```python
from build123d import *

# Parameters (mm, degrees)
F0_W     = 50.8
F0_H     = 19.05
F1_DEPTH = 1111.25
F2_W     = 122.435573
F2_H     = 50.8
F2_W_2   = 93.867282
F2_W_3   = 343.160421
F2_W_4   = 175.76392
F2_W_5   = 161.28926
F3_DEPTH = 25.4
F4_R     = 4.7625
F5_DEPTH = 25.4


with BuildPart() as f1:
    # F0 (on Top) → F1 (new body)
    with BuildSketch(Plane.XY):
        Rectangle(F0_W, F0_H)
    extrude(amount=F1_DEPTH)

    # F2 (on Front) → F3 (cut)
    with BuildSketch(Plane.XZ):
        with Locations((22.446524, 25.4)):
            Rectangle(F2_W, F2_H)
        with Locations((2.720783, 755.65)):
            Rectangle(F2_W_2, F2_H)
        with Locations((-38.781822, 1085.85)):
            Rectangle(F2_W_3, F2_H)
        with Locations((-28.949343, 254)):
            Rectangle(F2_W_4, F2_H)
        with Locations((-29.98326, 482.6)):
            Rectangle(F2_W_5, F2_H)
    extrude(amount=F3_DEPTH, mode=Mode.SUBTRACT)

    # F4 (on Front) → F5 (cut)
    with BuildSketch(Plane.XZ):
        with Locations((15.875, 254)):
            Circle(F4_R)
        with Locations((15.875, 482.6)):
            Circle(F4_R)
    extrude(amount=F5_DEPTH, mode=Mode.SUBTRACT)


solid = f1.part
```
Geometry: final body of the model. Coordinates: model frame, mm. A direction names the side the tool comes from. Coordinates: 2 decimals unless noted, no trailing zeros. Order: outer loops, then holes, each group sorted by start corner. A loop starts at its lowest first (then second) coordinate and runs counter-clockwise, first axis right, second up. Notation, with made-up numbers: M 33,47 L 44,47 A19 cw 44,59 Z; hole C 41,40.5 d8. An arc over 180 degrees is marked long. Answer as CSV lines item,"result".
Q1. First-contact query: P1, Ø5, axis at x = -6, y = -3.5, coming from the +Z side; P2, Ø3, axis at x = -4.5, y = -6, coming from the -Z side; P3, Ø15, axis at x = 9, z = 482, coming from the -Y side. Flat tips, straight axial feed; report the tip coordinate or a pass-through.
Answers:
P1,"stops at z = 1060.45"
P2,"stops at z = 50.8"
P3,"stops at y = 0"
Q2. Section B-B on x = 5.5. Return the cut outline in (y, z) (3 decimals).
Answers:
outline,"M -9.525,50.8 L 0,50.8 L 0,0 L 9.525,0 L 9.525,1111.25 L 0,1111.25 L 0,1060.45 L -9.525,1060.45 L -9.525,781.05 L 0,781.05 L 0,730.25 L -9.525,730.25 L -9.525,508 L 0,508 L 0,457.2 L -9.525,457.2 L -9.525,279.4 L 0,279.4 L 0,228.6 L -9.525,228.6 Z"
Q3. Section A-A on y = -3. Return the cut outline in (x, z), and give its area (3 significant figures).
Answers:
outline,"M -25.4,50.8 L 25.4,50.8 L 25.4,228.6 L -25.4,228.6 Z; M -25.4,279.4 L 25.4,279.4 L 25.4,457.2 L -25.4,457.2 Z; M -25.4,508 L 25.4,508 L 25.4,730.25 L -25.4,730.25 Z; M -25.4,781.05 L 25.4,781.05 L 25.4,1060.45 L -25.4,1060.45 Z"
area,"43,500 mm^2"
Q4. Draft query along Z for faces 1 (the flat face through (0, -9.525, 138)), 2 (the flat face through (0, 0, 756)). Return one class per face: pulls with the +Z half, pulls with the -Z half, needs draft (parallel to the pull), parting line crosses it, or undercut.
Answers:
face 1,"needs draft"
face 2,"undercut"
Q5. Set-up query: faces 3 (the flat face through (0, 0, 483)), 4 (the flat face through (0, 0, 26)), 5 (the flat face through (0, 0, 1086)), 6 (the flat face through (-25.4, 0, 548)), 7 (the flat face through (0, -9.525, 367)). Return all of +Z, -Z, +X, -X, +Y, -Y with unobstructed straight access to the full face (end or side cutting, diameter ignored); none if empty.
Answers:
face 3,"+X, -X, -Y"
face 4,"-Z, +X, -X, -Y"
face 5,"+Z, +X, -X, -Y"
face 6,"+Z, -Z, -X, +Y, -Y"
face 7,"+Z, -Z, +X, -X, -Y"
Q6. Section C-C on z = 262. Return the cut outline in (x, y) (3 decimals).
Answers:
outline,"M -25.4,0 L 25.4,0 L 25.4,9.525 L -25.4,9.525 Z"
Q7. Line query: probe 1 along Z at (x, y) = (0.5, -6). Output: solid intervals per line, ascending. Write a range as [from, to].
Answers:
probe 1,"z = [50.8, 228.6], [279.4, 457.2], [508, 730.25], [781.05, 1060.45]"
